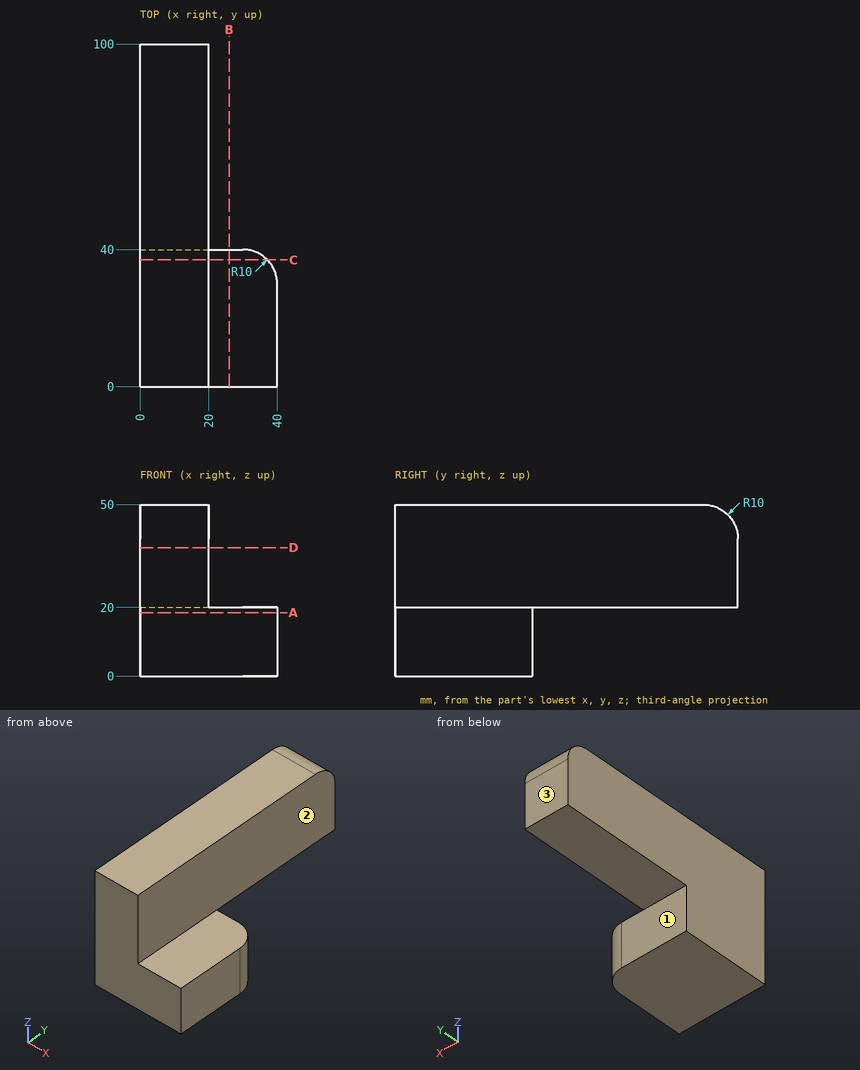
The drawing under review shows one solid part. Ordinate dimensions are in mm from its lowest x, y, z. A direction names the side the tool comes from. Round coordinates to 2 decimals unless told otherwise and drop trailing zeros. Loops run counter-clockwise (first coordinate to the right, second up) from the corner with the lowest first, then second, coordinate; pieces in that order, holes last. Notation, with made-up numbers: (39, -28) - (80, -28) arc R16 cw to (80, -16) - close; hole circle Ø5 at (25, -30.75). An arc over 180 degrees is marked (long way). Put each result on its own line as item: value. Start each with the question number.
1. Consider section C-C on y = 37. State the section outline as (x, z) points, plus the area to 3 significant figures.
2. Consider section A-A on z = 18.5. State the section outline as (x, y) points.
3. For the marked faces 1, 2 and 3, list the 3-axis set-ups (+Z, -Z, +X, -X, +Y, -Y) from which the entire face can be reached by the end or side of a thin tool; tool diameter is ignored.
4. Consider section D-D on z = 37.5. State the section outline as (x, y) points.
5. Consider section B-B on x = 26. State the section outline as (y, z) points.
6. For probe 1 along Z at (x, y) = (6.5, 51); probe 2 along X at (y, z) = (67, 34); probe 3 along Y at (x, z) = (25.5, 3.5), list the stretches that pass through material, from the lowest coordinate up. Write a range as [from, to].
7. Insertion check: P1, Ø9, axis at y = 51.5, z = 28, coming from the +X side; P2, Ø22, axis at x = 7, y = 84.5, coming from the -Z side; P3, Ø10, axis at x = 26, y = 19, coming from the +Z side. Each pin has a flat end and moves straight along its axis. Give the tip position at first contact, or say it passes through.
Result sheet:
1. outline: (0, 0) - (37.14, 0) - (37.14, 20) - (20, 20) - (20, 50) - (0, 50) - close
1. area: 1,340 mm^2
2. outline: (0, 0) - (40, 0) - (40, 30) arc R10 ccw to (30, 40) - (0, 40) - close
3. face 1: -Z, +X, -X, +Y
3. face 2: +Z, +X, +Y, -Y
3. face 3: +Z, -Z, +X, -X, +Y
4. outline: (0, 0) - (20, 0) - (20, 100) - (0, 100) - close
5. outline: (0, 0) - (40, 0) - (40, 20) - (0, 20) - close
6. probe 1: [20, 50]
6. probe 2: [0, 20]
6. probe 3: [0, 40]
7. P1: x = 20
7. P2: z = 20
7. P3: z = 20
